The listing builds one solid part. Answer for the finished solid, in the listing's coordinates (mm). A direction names the side the tool comes from. Give positions to 0.01 mm unless a question says otherwise; leave off trailing zeros. Write each loop counter-clockwise with the first axis right and the second up, starting at its lowest first coordinate (ties: lowest second). Pieces come first, ordered by that corner, then holes. Notation, with made-up numbers: (44.5, 31) -> (72.5, 31) arc R25 cw to (72.5, 44) -> close; hole circle Ø6 at (15, 66.5). An arc over 180 degrees is marked (long way). Use CSV: the item, a comma, the result in double quotes. Start each with the question number.
from build123d import *

# Parameters (mm, degrees)
SKETCH1_R           = 3.81
BOSS_EXTRUDE1_DEPTH = 32.1564
SKETCH2_R           = 1.9812
CUT_EXTRUDE1_DEPTH  = 33.604696916
SKETCH3_R           = 3.81
SKETCH3_R_2         = 3.429
CUT_EXTRUDE2_DEPTH  = 5.207
CUT_EXTRUDE3_START  = -9.652
SKETCH4_R           = 3.81
SKETCH4_R_2         = 3.556
CUT_EXTRUDE3_DEPTH  = 9.652
CHAMFER1_SIZE       = 0.508


with BuildPart() as part:
    # Sketch1 → Boss-Extrude1 (new body)
    with BuildSketch(Plane.XY):
        Circle(SKETCH1_R)
    extrude(amount=BOSS_EXTRUDE1_DEPTH)

    # Sketch2 → Cut-Extrude1 (cut, through all)
    with BuildSketch(Plane(origin=(0, 0, 0), x_dir=(-1, 0, 0), z_dir=(0, 0, -1))):
        Circle(SKETCH2_R)
    extrude(amount=-CUT_EXTRUDE1_DEPTH, mode=Mode.SUBTRACT)

    # Sketch3 → Cut-Extrude2 (cut)
    with BuildSketch(Plane(origin=(0, 0, 0), x_dir=(-1, 0, 0), z_dir=(0, 0, -1))):
        Circle(SKETCH3_R)
        Circle(SKETCH3_R_2, mode=Mode.SUBTRACT)
    extrude(amount=-CUT_EXTRUDE2_DEPTH, mode=Mode.SUBTRACT)

    # Sketch4 → Cut-Extrude3 (cut)
    with BuildSketch(Plane.XY.offset(32.1564).offset(CUT_EXTRUDE3_START)):
        with Locations(Location((0, 0, 0), (0, 0, 180))):
            Circle(SKETCH4_R)
        Circle(SKETCH4_R_2, mode=Mode.SUBTRACT)
    extrude(amount=CUT_EXTRUDE3_DEPTH, mode=Mode.SUBTRACT)

    # Sketch5 → Revolve1 (revolve)
    with BuildSketch(Plane(origin=(0, 0, 0), x_dir=(1, 0, 0), z_dir=(0, 1, 0))):
        with BuildLine():
            Line((3.556, -24.009676403), (3.269595119, -21.452809))
            Line((3.269595119, -21.452809), (3.81, -21.452809))
            ThreePointArc((3.81, -21.452809), (4.81966386, -22.844159242), (3.556, -24.009676403))
        make_face()
    revolve(axis=Axis((0, 0, 32.1564), (0, 0, -1)))

    # Chamfer1
    chamfer1_edges = [part.edges().sort_by_distance(p)[0] for p in [
        (-3.556, 0, 32.1564),
    ]]
    chamfer(chamfer1_edges, length=CHAMFER1_SIZE)


solid = part.part
Q1. Section A-A on x = 0 is taken. Give the vertices of the cut face in (y, z).
Q2. For faces 4 (the face through (-0.77, -3.47, 27.78)), 5 (the face through (0.74, -3.35, 2.57)), 6 (the face through (1, -2, 32.156)), determine the directions among +Z, -Z, +X, -X, +Y, -Y from which every point of the face is accessible in a straight line to the end or side of a thin tool.
Q3. Straight lines are drawn through the part: L1, parallel to Y at x = 0, z = 11.5; L2, parallel to Y at x = -3.25, z = 14; L3, parallel to X at y = -0.5, z = 27. For each, find the intervals that lie inside material, in ascending order.
Q4. Section C-C on z = 4 is taken. Give the vertices of the cut face in (x, y), then the cut area to 3 significant figures.
Q5. Section D-D on z = 25 is taken. Give the vertices of the cut face in (x, y), then the cut area to 3 significant figures.
Q6. Flat-ended cylindrical pins translate along their axes: pin 1 Ø1 at (x, z) = (-0.5, 4) entering from -Y; pin 2 Ø3 at (x, z) = (-2, 6) entering from +Y; pin 3 Ø1.5 at (x, z) = (1.5, 16.5) entering from +Y. Find the tip coordinate at first contact, or state that the pin passes through.
Q7. The mould has two halves that part along Y. Classify faces 1 (the face through (-0.83, -3.72, 13.22)), 2 (the face through (0.258, 1.964, 15.853)), 3 (the face through (3, 2, 5.207)): +Y half, -Y half, draft (parallel to the pull), parting line (faces both ways), or undercut.
Output:
1,outline,"(-3.81, 5.21) -> (-3.43, 5.21) -> (-3.43, 0) -> (-1.98, 0) -> (-1.98, 32.16) -> (-3.05, 32.16) -> (-3.56, 31.65) -> (-3.56, 24.01) arc R1.29 ccw to (-3.81, 21.45) -> close; (1.98, 0) -> (3.43, 0) -> (3.43, 5.21) -> (3.81, 5.21) -> (3.81, 21.45) arc R1.29 ccw to (3.56, 24.01) -> (3.56, 31.65) -> (3.05, 32.16) -> (1.98, 32.16) -> close"
2,face 4,"+Z"
2,face 5,"-Z"
2,face 6,"+Z, +X, -X, +Y, -Y"
3,L1,"-3.81 to -1.98, 1.98 to 3.81"
3,L2,"-1.99 to 1.99"
3,L3,"-3.52 to -1.92, 1.92 to 3.52"
4,outline,"circle Ø6.86 at (0, 0); hole circle Ø3.96 at (0, 0)"
4,area,"24.6 mm²"
5,outline,"circle Ø7.11 at (0, 0); hole circle Ø3.96 at (0, 0)"
5,area,"27.4 mm²"
6,pin 1,"y = -3.43"
6,pin 2,"y = 3.78"
6,pin 3,"y = 3.74"
7,face 1,"parting line"
7,face 2,"undercut"
7,face 3,"draft"
